Verification items for the finished model (mm, model axes). A direction names the side the tool comes from. Coordinates: 2 decimals unless noted, no trailing zeros. Order: outer loops, then holes, each group sorted by start corner. A loop starts at its lowest first (then second) coordinate and runs counter-clockwise, first axis right, second up.
Q1. Cross-section at A-A, the plane x = -93. Record the boundary of the cut face in (y, z), and give its area (3 significant figures).
Q2. Cross-section at D-D, the plane x = 0. Record the boundary of the cut face in (y, z), and give its area (3 significant figures).
Q3. Draft check along Z on faces 5 (the flat face through (74, 30, 0)), 6 (the flat face through (70, 30, 20)), 7 (the cylindrical face through (-103.58, 40.24, -62.17)). Enter one of: pulls with the +Z half, pulls with the -Z half, needs draft (parallel to the pull), parting line crosses it, or undercut.
Q4. Set-up check for faces 1 (the flat face through (-72, 101, -20)), 2 (the flat face through (-70, 10, 0)), 3 (the flat face through (-70, 60, 45)), 4 (the flat face through (-74, 42, -68)): record each of +Z, -Z, +X, -X, +Y, -Y from which the full face is reachable in a straight line by a thin tool's end or side.
Q5. Depth check by flat-ended pin: P1, Ø2.5, axis at x = -69, y = 45.5, coming from the -Z side; P2, Ø2.5, axis at x = -71, z = 37.5, coming from the +Y side; P3, Ø8, axis at x = -73, y = 105, coming from the -Z side; P4, Ø3, axis at y = 25, z = 21, coming from the +X side. Enter the tip coordinate at first touch or a pass-through.
Q6. Thickness scan on line 1 (X direction, y = 28.5, z = -1); line 2 (X direction, y = 24, z = -19); line 3 (X direction, y = 92, z = -4). Record the ranges inside material, lowest first.
Q7. Cross-section at C-C, the plane y = 134.5. Record the boundary of the cut face in (x, z), and give its area (3 significant figures).
Q8. Cross-section at B-B, the plane z = -38. Record the boundary of the cut face in (x, y), and give its area (3 significant figures).
from build123d import *

# Parameters (mm, degrees)
EXTRUDE_1_DEPTH     = 40
SKETCH_2_W          = 8
SKETCH_2_H          = 40
EXTRUDE_2_DEPTH     = 80
SKETCH_5_W          = 87.00766185
SKETCH_5_H          = 115.01495327
CUT_EXTRUDE_2_DEPTH = 10
SKETCH_6_R          = 85.063361003
CUT_EXTRUDE_3_DEPTH = 20
SKETCH_7_W          = 140
SKETCH_7_H          = 20
EXTRUDE_3_DEPTH     = 8
SKETCH_9_R          = 10
EXTRUDE_4_DEPTH     = 60
SKETCH_10_W         = 8
SKETCH_10_H         = 50
EXTRUDE_5_DEPTH     = 40
CUT_EXTRUDE_4_DEPTH = 40


with BuildPart() as part:
    # 草图1 → 凸台-拉伸1 (new body)
    with BuildSketch(Plane(origin=(0, 0, 0), x_dir=(1, 0, 0), z_dir=(0, 1, 0))):
        with BuildLine():
            Line((-74, 20), (-71.246052522, 20))
            ThreePointArc((-71.246052522, 20), (0, 74), (71.246052522, 20))
            Line((71.246052522, 20), (74, 20))
            Line((74, 20), (74, -20))
            Line((74, -20), (66, -20))
            Line((66, -20), (66, 0))
            ThreePointArc((66, 0), (0, 66), (-66, 0))
            Line((-66, 0), (-66, -20))
            Line((-66, -20), (-74, -20))
            Line((-74, -20), (-74, 20))
        make_face()
    extrude(amount=EXTRUDE_1_DEPTH)

    # 草图2 → 凸台-拉伸2 (add)
    with BuildSketch(Plane(origin=(0, 40, 0), x_dir=(1, 0, 0), z_dir=(0, 1, 0))):
        with Locations((-70, 0)):
            Rectangle(SKETCH_2_W, SKETCH_2_H)
        with Locations((70, 0)):
            Rectangle(SKETCH_2_W, SKETCH_2_H)
    extrude(amount=EXTRUDE_2_DEPTH)

    # 草图5 → 切除-拉伸2 (cut)
    with BuildSketch(Plane(origin=(74, 0, 0), x_dir=(0, 0, -1), z_dir=(1, 0, 0))):
        with Locations((-23.503830925, 97.507476635)):
            Rectangle(SKETCH_5_W, SKETCH_5_H)
    extrude(amount=-CUT_EXTRUDE_2_DEPTH, mode=Mode.SUBTRACT)

    # 草图6 → 切除-拉伸3 (cut)
    with BuildSketch(Plane.XZ):
        Circle(SKETCH_6_R)
        with BuildLine():
            Line((-71.246052522, 20), (-66, 20))
            Line((-66, 20), (-66, 0))
            Line((-66, 0), (-74, 0))
            ThreePointArc((-74, 0), (0, -74), (74, 0))
            Line((74, 0), (66, 0))
            Line((66, 0), (66, 20))
            Line((66, 20), (71.246052522, 20))
            ThreePointArc((71.246052522, 20), (0, 74), (-71.246052522, 20))
        make_face(mode=Mode.SUBTRACT)
    extrude(amount=-CUT_EXTRUDE_3_DEPTH, mode=Mode.SUBTRACT)

    # 草图7 → 凸台-拉伸3 (add)
    with BuildSketch(Plane.ZY.offset(74)):
        with Locations((0, 50)):
            Rectangle(SKETCH_7_W, SKETCH_7_H)
    extrude(amount=-EXTRUDE_3_DEPTH)

    # 草图9 → 凸台-拉伸4 (add)
    with BuildSketch(Plane.ZY.offset(74)):
        with Locations((-60, 50)):
            Circle(SKETCH_9_R)
        with Locations((60, 50)):
            Circle(SKETCH_9_R)
    extrude(amount=EXTRUDE_4_DEPTH)

    # 草图10 → 凸台-拉伸5 (add)
    with BuildSketch(Plane.XY.offset(20)):
        with Locations((-78, 135)):
            Rectangle(SKETCH_10_W, SKETCH_10_H)
    extrude(amount=-EXTRUDE_5_DEPTH)

    # 草图11 → 切除-拉伸4 (cut)
    with BuildSketch(Plane.ZY.offset(82)):
        with BuildLine():
            Line((-20, 140), (-20, 168.258518719))
            Line((-20, 168.258518719), (20, 168.258518719))
            Line((20, 168.258518719), (20, 140))
            ThreePointArc((20, 140), (0, 160), (-20, 140))
        make_face()
    extrude(amount=-CUT_EXTRUDE_4_DEPTH, mode=Mode.SUBTRACT)


solid = part.part
Check values:
1. outline: circle Ø20 at (50, -60); circle Ø20 at (50, 60)
1. area: 628 mm2
2. outline: (0, -74) - (40, -74) - (40, -66) - (0, -66) - close
2. area: 320 mm2
3. face 5: needs draft
3. face 6: pulls with the +Z half
3. face 7: undercut
4. face 1: -Z, +X, -X, +Y
4. face 2: +Z, +X, -X, -Y
4. face 3: +Z, +X, -X, +Y
4. face 4: -Z, -X, -Y
5. P1: stops at z = -70
5. P2: stops at y = 60
5. P3: stops at z = -20
5. P4: stops at x = 74
6. line 1: x = -74 to -65.99, 65.99 to 74
6. line 2: x = -74 to -63.21, 63.21 to 74
6. line 3: x = -74 to -66
7. outline: (-82, -20) - (-74, -20) - (-74, 20) - (-82, 20) - close
7. area: 320 mm2
8. outline: (-74, 40) - (-66, 40) - (-66, 60) - (-74, 60) - close; (-63.5, 0) - (-53.96, 0) - (-53.96, 40) - (-63.5, 40) - close; (53.96, 0) - (63.5, 0) - (63.5, 40) - (53.96, 40) - close
8. area: 923 mm2
